Work out the finished part from the listing and answer in its coordinate system (mm). A direction names the side the tool comes from. Round coordinates to 2 decimals unless told otherwise and drop trailing zeros. Order: outer loops, then holes, each group sorted by start corner. A loop starts at its lowest first (then second) coordinate and runs counter-clockwise, first axis right, second up. Notation, with made-up numbers: (-31, 49.5) - (15, 49.5) arc R20 cw to (15, 69.5) - close; hole circle Ø10 at (42, 21.25). An arc over 180 degrees is marked (long way). Answer in a Markdown table with one row per item.
from build123d import *

# Parameters (mm, degrees)
SKETCH1_W           = 50
SKETCH1_H           = 50
BOSS_EXTRUDE1_DEPTH = 300
SKETCH2_R           = 7.5
CUT_EXTRUDE1_DEPTH  = 15


with BuildPart() as part:
    # Sketch1 → Boss-Extrude1 (new body)
    with BuildSketch(Plane.XY):
        with Locations((475, -275)):
            Rectangle(SKETCH1_W, SKETCH1_H)
    extrude(amount=BOSS_EXTRUDE1_DEPTH)

    # Sketch2 → Cut-Extrude1 (cut)
    with BuildSketch(Plane(origin=(0, -250, 0), x_dir=(1, 0, 0), z_dir=(0, 1, 0))):
        with Locations((475, -150)):
            Circle(SKETCH2_R)
    extrude(amount=-CUT_EXTRUDE1_DEPTH, mode=Mode.SUBTRACT)


solid = part.part
1) The mould has two halves that part along X. Classify faces 1 (the face through (464, -250, 148)), 2 (the face through (475, -265, 150)), 3 (the face through (500, -275, 148)): released by +X, released by -X, zero draft, split by the parting line, or undercut.
Filled in:
| item | result |
|---|---|
| face 1 | zero draft |
| face 2 | undercut |
| face 3 | released by +X |
2) Find the intervals of material crossed by probe 1 along Z at (x, y) = (475, -261); probe 2 along X at (y, z) = (-253.75, 150); probe 3 along Z at (x, y) = (470, -257.5), in increasing order. Write a range as from..to.
Filled in:
| item | result |
|---|---|
| probe 1 | z = 0..142.5, 157.5..300 |
| probe 2 | x = 450..467.5, 482.5..500 |
| probe 3 | z = 0..144.41, 155.59..300 |
3) Which of the six approach directions +Z, -Z, +X, -X, +Y, -Y give full straight-line access (tool end or side, diameter ignored) to faces 4 (the face through (475, -275, 0)), 5 (the face through (482.154, -257.395, 147.747))?
Filled in:
| item | result |
|---|---|
| face 4 | -Z, +X, -X, +Y, -Y |
| face 5 | +Y |
4) Find section A-A, the plane x = 475. Give the vertices of the cut face in (y, z), then the cut area to 3 significant figures.
Filled in:
| item | result |
|---|---|
| outline | (-300, 0) - (-250, 0) - (-250, 142.5) - (-265, 142.5) - (-265, 157.5) - (-250, 157.5) - (-250, 300) - (-300, 300) - close |
| area | 14,800 mm^2 |
5) This flat-tipped pin is pushed along its axis until it touches: pin 1 (7.5 mm diameter, centred on x = 477.5, z = 147.5, fed in from +Y). Where does it stop, or does it pass through?
Filled in:
| item | result |
|---|---|
| pin 1 | stops at y = -265 |
6) Find section B-B, the plane z = 150. Give the vertices of the cut face in (x, y).
Filled in:
| item | result |
|---|---|
| outline | (450, -300) - (500, -300) - (500, -250) - (482.5, -250) - (482.5, -265) - (467.5, -265) - (467.5, -250) - (450, -250) - close |
